from build123d import *

# Parameters (mm, degrees)
BASE_FLANGE1_DEPTH           = 448.31
CUT_EXTRUDE1_DEPTH           = 459.458977562
F_1_4_CLEARANCE_HOLE1_D      = 6.7564
F_10_0_1935_DIAMETER_HOLE1_D = 4.9149
CUT_EXTRUDE2_DEPTH           = 459.458977562
FILLET1_R                    = 3.81


# Sheet-metal steps are written as plain solids
with BuildPart() as part:
    # Sketch2 → Base-Flange1 (new body)
    with BuildSketch(Plane(origin=(0, 0, 0), x_dir=(0, 0, -1), z_dir=(1, 0, 0))):
        with BuildLine():
            Line((-40.68826, -50.8), (-40.68826, -5.76326))
            ThreePointArc((-40.68826, -5.76326), (-39.000240228, -1.688019772), (-34.925, 0))
            Line((-34.925, 0), (34.925, 0))
            ThreePointArc((34.925, 0), (39.000240228, -1.688019772), (40.68826, -5.76326))
            Line((40.68826, -5.76326), (40.68826, -50.8))
            Line((40.68826, -50.8), (38.1, -50.8))
            Line((38.1, -50.8), (38.1, -5.76326))
            ThreePointArc((38.1, -5.76326), (37.17006403, -3.51819597), (34.925, -2.58826))
            Line((34.925, -2.58826), (-34.925, -2.58826))
            ThreePointArc((-34.925, -2.58826), (-37.17006403, -3.51819597), (-38.1, -5.76326))
            Line((-38.1, -5.76326), (-38.1, -50.8))
            Line((-38.1, -50.8), (-40.68826, -50.8))
        make_face()
    extrude(amount=BASE_FLANGE1_DEPTH)

    # Sketch8 → Cut-Extrude1 (cut, through all)
    with BuildSketch(Plane.XY.offset(40.68826)):
        Polygon((0, -37.636171444), (49.128076995, -50.8), (0, -50.8), align=None)
    extrude(amount=-CUT_EXTRUDE1_DEPTH, mode=Mode.SUBTRACT)

    # 1/4 Clearance Hole1 (through all)
    with Locations(Plane.XY.offset(40.68826)):
        with Locations((8.61046841, -16.934326391)):
            Hole(F_1_4_CLEARANCE_HOLE1_D / 2)

    # #10 (0.1935) Diameter Hole1 (through all)
    with Locations(Plane.XY.offset(40.68826)):
        with Locations((410.50096824, -26.010505082), (413.952320207, -13.129884188), (436.899172539, -13.361871369), (431.968669729, -31.762758359), (39.880176489, -35.174025037), (45.632429766, -13.706323547), (85.501018246, -24.389079634), (134.570050222, -37.537087125)):
            Hole(F_10_0_1935_DIAMETER_HOLE1_D / 2)

    # Sketch9 → Cut-Extrude2 (cut, through all)
    with BuildSketch(Plane.XY.offset(40.68826)):
        Polygon((140.864867564, -75.380798949), (152.369374119, -32.445395971), (220.869688909, -50.8), (209.365182354, -93.735402979), align=None)
    extrude(amount=-CUT_EXTRUDE2_DEPTH, mode=Mode.SUBTRACT)

    # Fillet1
    fillet1_edges = [part.edges().sort_by_distance(p)[0] for p in [
        (147.451272792, -50.8, -39.39413),
        (147.451272792, -50.8, 39.39413),
        (152.369374119, -32.445395971, -39.39413),
        (152.369374119, -32.445395971, 39.39413),
        (220.869688909, -50.8, -39.39413),
        (220.869688909, -50.8, 39.39413),
        (448.31, -50.8, 39.39413),
        (49.128076995, -50.8, -39.39413),
        (0, -37.636171444, -39.39413),
        (0, -37.636171444, 39.39413),
        (49.128076995, -50.8, 39.39413),
        (448.31, -50.8, -39.39413),
    ]]
    fillet(fillet1_edges, radius=FILLET1_R)


solid = part.part
Input: part model. Units: mm. Frame: model coordinates. A direction names the side the tool comes from. Give positions to 0.01 mm unless a question says otherwise; leave off trailing zeros. Loops run counter-clockwise (first coordinate to the right, second up) from the corner with the lowest first, then second, coordinate; pieces in that order, holes last. Notation, with made-up numbers: (31, -22) - (58, -22) arc R20 ccw to (58, -3) - close; hole circle Ø8 at (5, 44). An arc over 180 degrees is marked (long way). Use CSV: the item, a comma, the result in double quotes. Start each with the question number.
Item 1: Mould query, pull axis X, two halves, no side actions, for faces 3 (the flat face through (25.413, -44.446, 39.412)), 4 (the flat face through (187.77, -41.93, 39.41)), 5 (the flat face through (187.77, -41.93, -39.38)), 6 (the flat face through (221, -29, 40.688)). Classes: pulls with the +X half, pulls with the -X half, needs draft (parallel to the pull), parting line crosses it, or undercut.
Item 2: Line query: line 1 (Z direction, x = 56, y = -12.5); line 2 (Y direction, x = 246, z = -16.5); line 3 (Y direction, x = 40, z = -36.5). Output: solid intervals per line, ascending.
Item 3: Section C-C on x = 212. Return loops of the section in (y, z) (3 decimals).
Item 4: Reachability of faces 1 (the flat face through (221, -28, 38.1)), 2 (the flat face through (448.31, -1, 0)) from +Z, -Z, +X, -X, +Y, -Y: full face, straight path, thin tool, end or side. Return the list, or none.
Item 5: Contact query for a flat-ended pin moving along its axis: P1, Ø1, axis at x = 119, z = -28.5, coming from the -Y side. Output: stop coordinate, or through.
Item 6: Section B-B on z = 23. Return loops of the section in (x, y).
Item 7: Section A-A on x = 59.5. Return loops of the section in (y, z) (3 decimals).
Ans:
1,face 3,"pulls with the -X half"
1,face 4,"undercut"
1,face 5,"undercut"
1,face 6,"needs draft"
2,line 1,"z = -40.69 to -38.1, 38.1 to 40.69"
2,line 2,"y = -2.59 to 0"
2,line 3,"y = -3.01 to -0.22"
3,outline,"(-48.423, -40.688) - (-5.763, -40.688) arc R5.763 ccw to (0, -34.925) - (0, 34.925) arc R5.763 ccw to (-5.763, 40.688) - (-48.423, 40.688) - (-48.423, 38.1) - (-5.763, 38.1) arc R3.175 cw to (-2.588, 34.925) - (-2.588, -34.925) arc R3.175 cw to (-5.763, -38.1) - (-48.423, -38.1) - close"
4,face 1,"+X, -X, -Y"
4,face 2,"+Z, -Z, +X, +Y, -Y"
5,P1,"stops at y = -2.59"
6,outline,"(0, -2.59) - (448.31, -2.59) - (448.31, 0) - (0, 0) - close"
7,outline,"(-50.8, -40.688) - (-5.763, -40.688) arc R5.763 ccw to (0, -34.925) - (0, 34.925) arc R5.763 ccw to (-5.763, 40.688) - (-50.8, 40.688) - (-50.8, 38.1) - (-5.763, 38.1) arc R3.175 cw to (-2.588, 34.925) - (-2.588, -34.925) arc R3.175 cw to (-5.763, -38.1) - (-50.8, -38.1) - close"
